Model file for the job. Use its own axes, mm. Face numbers are marked on the shaded views. A direction names the side the tool comes from. Coordinates: 2 decimals unless noted, no trailing zeros. Order: outer loops, then holes, each group sorted by start corner. A loop starts at its lowest first (then second) coordinate and runs counter-clockwise, first axis right, second up. Notation, with made-up numbers: (45.5, 4) -> (76.5, 4) arc R36 cw to (76.5, 40) -> close; hole circle Ø6 at (69, 28.25). An arc over 180 degrees is marked (long way). Return JSON: item names as keys, results as strings. Group by question number.
1) Cut at D-D (y = -1.5). Write the cut outline in (x, z).
2) Probe line 1 (Z direction, x = -7, y = 31); line 2 (Z direction, x = -17, y = 34); line 3 (Z direction, x = -48, y = 2). List the from-to ranges inside material, lowest first.
3) Cut at C-C (z = 18). Write the cut outline in (x, y).
4) Pull direction Z, two halves, no side cores. Call the marked faces 1, 2 and 3: +Z half, -Z half, draft (parallel to the pull), parting line (faces both ways), or undercut.
5) Which spindle directions (+Z, -Z, +X, -X, +Y, -Y) get a long thin tool onto all of the face, cutting with end or side? Do the marked faces 4, 5, 6, 7 and 8. Say none if no direction does.
6) Cut at A-A (y = -24.5). Write the cut outline in (x, z), and give its area (3 significant figures).
7) Flat gauge pins, fed straight in: pin 1 (4 mm diameter, centred on x = -6, z = 11.5, fed in from -Y); pin 2 (6 mm diameter, centred on y = 25.5, z = 10.5, fed in from +X); pin 3 (8 mm diameter, centred on x = -30.5, y = -22.5, fed in from -Z). Where does each tip first touch, or does it go through?
8) Cut at B-B (x = 10). Write the cut outline in (y, z).
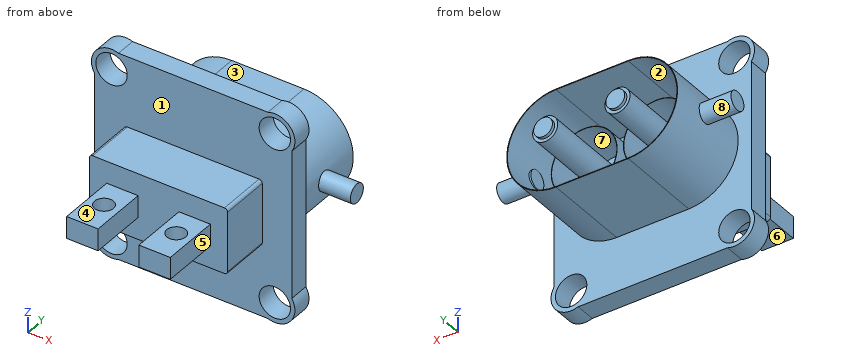
from build123d import *

# Parameters (mm, degrees)
DODANIE_WYCI_GNI_CIE1_DEPTH      = 6.5
SZKIC2_R                         = 6.4
DODANIE_WYCI_GNI_CIE2_DEPTH      = 6.5
SZKIC3_R                         = 5
WYTNIJ_WYCI_GNI_CIE4_DEPTH       = 6.5
SZKIC4_R                         = 10.5
SZKIC4_R_2                       = 10.4
DODANIE_WYCI_GNI_CIE3_DEPTH      = 15
DODANIE_WYCI_GNI_CIE4_DEPTH      = 16
SZKIC6_W                         = 10
SZKIC6_H                         = 7
DODANIE_WYCI_GNI_CIE5_DEPTH      = 34.5
SZKIC7_R                         = 4
DODANIE_WYCI_GNI_CIE6_DEPTH      = 33
SZKIC8_R                         = 3
DODANIE_WYCI_GNI_CIE7_DEPTH      = 1
SZKIC9_R                         = 3
DODANIE_WYCI_GNI_CIE8_DEPTH      = 5.9
DODANIE_WYCI_GNI_CIE8_DEPTH_BACK = 5
SZKIC10_R                        = 3
DODANIE_WYCI_GNI_CIE9_DEPTH      = 5.9
DODANIE_WYCI_GNI_CIE9_DEPTH_BACK = 5
DODANIE_WYCI_GNI_CIE10_DEPTH     = 28
SZKIC12_R                        = 3
WYTNIJ_WYCI_GNI_CIE5_DEPTH       = 7


with BuildPart() as part:
    # Szkic1 → Dodanie-wyci_gni_cie1 (new body)
    with BuildSketch(Plane(origin=(0, 0, 0), x_dir=(1, 0, 0), z_dir=(0, 1, 0))):
        with BuildLine():
            Line((-49.920411058, 35.319148676), (-49.920411058, -21.880851324))
            ThreePointArc((-49.920411058, -21.880851324), (-48.631680895, -24.992121161), (-45.520411058, -26.280851324))
            Line((-45.520411058, -26.280851324), (8.479588942, -26.280851324))
            ThreePointArc((8.479588942, -26.280851324), (11.590858779, -24.992121161), (12.879588942, -21.880851324))
            Line((12.879588942, -21.880851324), (12.879588942, 35.319148676))
            ThreePointArc((12.879588942, 35.319148676), (11.590858779, 38.430418513), (8.479588942, 39.719148676))
            Line((8.479588942, 39.719148676), (-45.520411058, 39.719148676))
            ThreePointArc((-45.520411058, 39.719148676), (-48.631680895, 38.430418513), (-49.920411058, 35.319148676))
        make_face()
    extrude(amount=DODANIE_WYCI_GNI_CIE1_DEPTH)

    # Szkic2 → Dodanie-wyci_gni_cie2 (add)
    with BuildSketch(Plane(origin=(0, 0, 0), x_dir=(1, 0, 0), z_dir=(0, 1, 0))):
        with Locations((-44.520411058, 33.719148676)):
            Circle(SZKIC2_R)
        with Locations((-44.520411058, -20.280851324)):
            Circle(SZKIC2_R)
        with Locations((7.479588942, -20.280851324)):
            Circle(SZKIC2_R)
        with Locations((7.479588942, 33.719148676)):
            Circle(SZKIC2_R)
    extrude(amount=DODANIE_WYCI_GNI_CIE2_DEPTH)

    # Szkic3 → Wytnij-wyci_gni_cie4 (cut)
    with BuildSketch(Plane(origin=(0, 6.5, 0), x_dir=(1, 0, 0), z_dir=(0, 1, 0))):
        with Locations((7.479588942, 33.719148676)):
            Circle(SZKIC3_R)
        with Locations((-44.520411058, 33.719148676)):
            Circle(SZKIC3_R)
        with Locations((7.479588942, -20.280851324)):
            Circle(SZKIC3_R)
        with Locations((-44.520411058, -20.280851324)):
            Circle(SZKIC3_R)
    extrude(amount=-WYTNIJ_WYCI_GNI_CIE4_DEPTH, mode=Mode.SUBTRACT)

    # Szkic4 → Dodanie-wyci_gni_cie3 (add)
    with BuildSketch(Plane(origin=(0, 6.5, 0), x_dir=(1, 0, 0), z_dir=(0, 1, 0))):
        with Locations((-30.020411058, 6.719148676)):
            Circle(SZKIC4_R)
        with Locations((-30.020411058, 6.719148676)):
            Circle(SZKIC4_R_2, mode=Mode.SUBTRACT)
        with Locations((-7.020411058, 6.719148676)):
            Circle(SZKIC4_R)
        with Locations((-7.020411058, 6.719148676)):
            Circle(SZKIC4_R_2, mode=Mode.SUBTRACT)
    extrude(amount=DODANIE_WYCI_GNI_CIE3_DEPTH)

    # Szkic5 → Dodanie-wyci_gni_cie4 (add)
    with BuildSketch(Plane(origin=(0, 0, 0), x_dir=(-1, 0, 0), z_dir=(0, -1, 0))):
        with BuildLine():
            Line((-3.479588942, -2.780851324), (-3.479588942, 16.219148676))
            ThreePointArc((-3.479588942, 16.219148676), (-3.186695723, 16.926255457), (-2.479588942, 17.219148676))
            Line((-2.479588942, 17.219148676), (39.520411058, 17.219148676))
            ThreePointArc((39.520411058, 17.219148676), (40.227517839, 16.926255457), (40.520411058, 16.219148676))
            Line((40.520411058, 16.219148676), (40.520411058, -2.780851324))
            ThreePointArc((40.520411058, -2.780851324), (40.227517839, -3.487958105), (39.520411058, -3.780851324))
            Line((39.520411058, -3.780851324), (-2.479588942, -3.780851324))
            ThreePointArc((-2.479588942, -3.780851324), (-3.186695723, -3.487958105), (-3.479588942, -2.780851324))
        make_face()
    extrude(amount=DODANIE_WYCI_GNI_CIE4_DEPTH)

    # Szkic6 → Dodanie-wyci_gni_cie5 (add)
    with BuildSketch(Plane(origin=(0, 0, 0), x_dir=(-1, 0, 0), z_dir=(0, -1, 0))):
        with Locations((30.020411058, 6.719148676)):
            Rectangle(SZKIC6_W, SZKIC6_H)
        with Locations((7.020411058, 6.719148676)):
            Rectangle(SZKIC6_W, SZKIC6_H)
    extrude(amount=DODANIE_WYCI_GNI_CIE5_DEPTH)

    # Szkic7 → Dodanie-wyci_gni_cie6 (add)
    with BuildSketch(Plane(origin=(0, 6.5, 0), x_dir=(1, 0, 0), z_dir=(0, 1, 0))):
        with Locations((-30.020411058, 6.719148676)):
            Circle(SZKIC7_R)
        with Locations((-7.020411058, 6.719148676)):
            Circle(SZKIC7_R)
    extrude(amount=DODANIE_WYCI_GNI_CIE6_DEPTH)

    # Szkic8 → Dodanie-wyci_gni_cie7 (add)
    with BuildSketch(Plane(origin=(0, 39.5, 0), x_dir=(1, 0, 0), z_dir=(0, 1, 0))):
        with Locations((-30.020411058, 6.719148676)):
            Circle(SZKIC8_R)
        with Locations((-7.020411058, 6.719148676)):
            Circle(SZKIC8_R)
    extrude(amount=DODANIE_WYCI_GNI_CIE7_DEPTH)



with BuildPart() as body_2:
    # Szkic9 → Dodanie-wyci_gni_cie8 (new body, two sides)
    with BuildSketch(Plane.ZY.offset(49.920411058)) as dodanie_wyci_gni_cie8_sk:
        with Locations((-6.719148676, 21.5)):
            Circle(SZKIC9_R)
    extrude(amount=DODANIE_WYCI_GNI_CIE8_DEPTH)
    extrude(dodanie_wyci_gni_cie8_sk.sketch, amount=-DODANIE_WYCI_GNI_CIE8_DEPTH_BACK)


with BuildPart() as body_3:
    # Szkic10 → Dodanie-wyci_gni_cie9 (new body, two sides)
    with BuildSketch(Plane(origin=(12.879588942, 0, 0), x_dir=(0, 0, -1), z_dir=(1, 0, 0))) as dodanie_wyci_gni_cie9_sk:
        with Locations((6.719148676, 21.5)):
            Circle(SZKIC10_R)
    extrude(amount=DODANIE_WYCI_GNI_CIE9_DEPTH)
    extrude(dodanie_wyci_gni_cie9_sk.sketch, amount=-DODANIE_WYCI_GNI_CIE9_DEPTH_BACK)


with BuildPart() as part_1:
    add(part.part)

    add(body_2.part)  # Dodanie-wyci_gni_cie10 merges body 2

    add(body_3.part)  # Dodanie-wyci_gni_cie10 merges body 3
    # Szkic11 → Dodanie-wyci_gni_cie10 (add)
    with BuildSketch(Plane(origin=(0, 6.5, 0), x_dir=(1, 0, 0), z_dir=(0, 1, 0))):
        with BuildLine():
            Line((-7.020411058, 22.419148676), (-30.020411058, 22.419148676))
            ThreePointArc((-30.020411058, 22.419148676), (-45.720411058, 6.719148676), (-30.020411058, -8.980851324))
            Line((-30.020411058, -8.980851324), (-7.020411058, -8.980851324))
            ThreePointArc((-7.020411058, -8.980851324), (8.679588942, 6.719148676), (-7.020411058, 22.419148676))
        make_face()
        with BuildLine():
            Line((-7.020411058, 22.219148676), (-30.020411058, 22.219148676))
            ThreePointArc((-30.020411058, 22.219148676), (-45.520411058, 6.719148676), (-30.020411058, -8.780851324))
            Line((-30.020411058, -8.780851324), (-7.020411058, -8.780851324))
            ThreePointArc((-7.020411058, -8.780851324), (8.479588942, 6.719148676), (-7.020411058, 22.219148676))
        make_face(mode=Mode.SUBTRACT)
    extrude(amount=DODANIE_WYCI_GNI_CIE10_DEPTH)

    # Szkic12 → Wytnij-wyci_gni_cie5 (cut)
    with BuildSketch(Plane.XY.offset(-3.219148676)):
        with Locations((-7.020411058, -24.5)):
            Circle(SZKIC12_R)
        with Locations((-30.020411058, -24.5)):
            Circle(SZKIC12_R)
    extrude(amount=-WYTNIJ_WYCI_GNI_CIE5_DEPTH, mode=Mode.SUBTRACT)


solid = part_1.part
Answers below:
{
 "1": {"outline": "(-40.52, -16.22) arc R1 ccw to (-39.52, -17.22) -> (2.48, -17.22) arc R1 ccw to (3.48, -16.22) -> (3.48, 2.78) arc R1 ccw to (2.48, 3.78) -> (-39.52, 3.78) arc R1 ccw to (-40.52, 2.78) -> close"},
 "2": {"line 1": "z = -22.42 to -22.22, -10.72 to -2.72, 8.78 to 8.98", "line 2": "z = -22.42 to -22.22, 8.78 to 8.98", "line 3": "z = -39.09 to -37.31, -30.13 to 16.69, 23.87 to 25.65"},
 "3": {"outline": "(-50.5, 0) -> (-48.97, 0) -> (-48.97, 6.5) -> (-50.5, 6.5) -> close; (-40.07, 0) -> (3.03, 0) -> (3.03, 6.5) -> (-40.07, 6.5) -> close; (11.93, 0) -> (13.46, 0) -> (13.46, 6.5) -> (11.93, 6.5) -> close"},
 "4": {"face 1": "draft", "face 2": "undercut", "face 3": "+Z half"},
 "5": {"face 4": "+Z, +X, -X, -Y", "face 5": "+Z, -Z, +X, -Y", "face 6": "-Z, +X, -X, -Y", "face 7": "+Y", "face 8": "-X"},
 "6": {"outline": "(-35.02, -10.22) -> (-33.02, -10.22) -> (-33.02, -3.22) -> (-35.02, -3.22) -> close; (-27.02, -10.22) -> (-25.02, -10.22) -> (-25.02, -3.22) -> (-27.02, -3.22) -> close; (-12.02, -10.22) -> (-10.02, -10.22) -> (-10.02, -3.22) -> (-12.02, -3.22) -> close; (-4.02, -10.22) -> (-2.02, -10.22) -> (-2.02, -3.22) -> (-4.02, -3.22) -> close", "area": "56.0 mm^2"},
 "7": {"pin 1": "stops at y = 0", "pin 2": "stops at x = -0.36", "pin 3": "stops at z = -10.22"},
 "8": {"outline": "(0, -39.6) -> (6.5, -39.6) -> (6.5, -38.04) -> (0, -38.04) -> close; (0, -29.4) -> (6.5, -29.4) -> (6.5, 15.96) -> (0, 15.96) -> close; (0, 24.6) -> (6.5, 24.6) -> (6.5, 26.16) -> (0, 26.16) -> close; circle Ø6 at (21.5, -6.72)"}
}
